from build123d import *

# Parameters (mm, degrees)
EXTRUDE_1_DEPTH     = 16.5
CUT_EXTRUDE_1_DEPTH = 89.239730281
SKETCH_3_R          = 3
CUT_EXTRUDE_2_DEPTH = 33


with BuildPart() as part:
    # 草圖1 → 填料-伸長1 (new, symmetric)
    with BuildSketch(Plane.XY):
        Polygon((0, 0), (85, 0), (85, 10), (78, 10), (78, 17), (75.5, 17), (75.5, 23), (63.5, 23), (63.5, 17), (61, 17), (61, 10), (50, 10), (50, 6), (0, 6), align=None)
    extrude(amount=EXTRUDE_1_DEPTH, both=True)

    # 草圖2 → 除料-伸長1 (cut, through all)
    with BuildSketch(Plane(origin=(0, 6, 0), x_dir=(1, 0, 0), z_dir=(0, 1, 0))):
        with BuildLine():
            Line((10, 4), (45, 4))
            ThreePointArc((45, 4), (49, 0), (45, -4))
            Line((45, -4), (10, -4))
            ThreePointArc((10, -4), (6, 0), (10, 4))
        make_face()
    extrude(amount=-CUT_EXTRUDE_1_DEPTH, mode=Mode.SUBTRACT)

    # 草圖3 → 除料-伸長2 (cut)
    with BuildSketch(Plane(origin=(78, 0, 0), x_dir=(0, 0, -1), z_dir=(1, 0, 0))):
        with Locations(Location((-10, 15, 0), (0, 0, 41.810314896))):
            Circle(SKETCH_3_R)
        with Locations(Location((10, 15, 0), (0, 0, 41.810314896))):
            Circle(SKETCH_3_R)
    extrude(amount=-CUT_EXTRUDE_2_DEPTH, mode=Mode.SUBTRACT)


solid = part.part
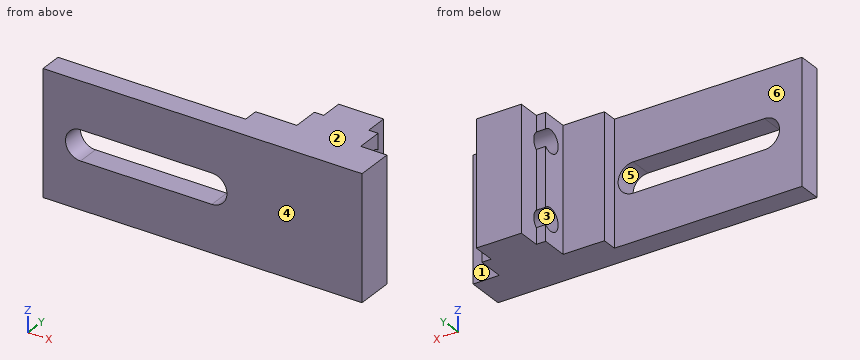
Can you work these out from the model? Positions are in its coordinate system, mm. Face numbers are marked on the shaded views. A direction names the side the tool comes from. Round coordinates to 2 decimals unless told otherwise and drop trailing zeros. Order: outer loops, then holes, each group sorted by start corner. A loop starts at its lowest first (then second) coordinate and runs counter-clockwise, first axis right, second up. Notation, with made-up numbers: (-9.75, 20.5) - (2.25, 20.5) arc R31 ccw to (2.25, 54.5) - close; hole circle Ø2 at (57, -8.75). An arc over 180 degrees is marked (long way). Answer in a Markdown table with one row per item.
(1) Suppose I cut it at B-B, the plane x = 14. Please give me the cut outline in (y, z).
From the geometry:
| item | result |
|---|---|
| outline | (0, -16.5) - (6, -16.5) - (6, -4) - (0, -4) - close; (0, 4) - (6, 4) - (6, 16.5) - (0, 16.5) - close |
(2) Suppose I cut it at A-A, the plane z = -10. Please give me the cut outline in (x, y), plus the area to 3 significant figures.
From the geometry:
| item | result |
|---|---|
| outline | (0, 0) - (85, 0) - (85, 10) - (78, 10) - (78, 12) - (61, 12) - (61, 10) - (50, 10) - (50, 6) - (0, 6) - close; (63.5, 18) - (75.5, 18) - (75.5, 23) - (63.5, 23) - close |
| area | 744 mm2 |
(3) Suppose I cut it at D-D, the plane x = 70.5. Please give me the cut outline in (y, z), plus the area to 3 significant figures.
From the geometry:
| item | result |
|---|---|
| outline | (0, -16.5) - (23, -16.5) - (23, 16.5) - (0, 16.5) - close; hole circle Ø6 at (15, -10); hole circle Ø6 at (15, 10) |
| area | 702 mm2 |
(4) Suppose I cut it at C-C, the plane y = 15. Please give me the cut outline in (x, z), plus the area to 3 significant figures.
From the geometry:
| item | result |
|---|---|
| outline | (61, -16.5) - (78, -16.5) - (78, -13) - (61, -13) - close; (61, -7) - (78, -7) - (78, 7) - (61, 7) - close; (61, 13) - (78, 13) - (78, 16.5) - (61, 16.5) - close |
| area | 357 mm2 |
(5) Please list where these lines run through material, in increasing order: L1, parallel to Z at x = 65, y = 15; L2, parallel to Y at x = 68, z = 10; L3, parallel to Z at x = 15, y = 5.25. Write a range as from..to.
From the geometry:
| item | result |
|---|---|
| L1 | z = -16.5..-13, -7..7, 13..16.5 |
| L2 | y = 0..12, 18..23 |
| L3 | z = -16.5..-4, 4..16.5 |
(6) Which directions (+Z, -Z, +X, -X, +Y, -Y) give clear straight access to the entire face, cutting with the end or side of a thin tool? Please do the marked faces 4, 5 and 6.
From the geometry:
| item | result |
|---|---|
| face 4 | +Z, -Z, +X, -X, -Y |
| face 5 | +Y, -Y |
| face 6 | +Z, -Z, -X, +Y |
(7) If we mould it in two halves opening along Y, with no side actions, what happens to the marked faces 1, 2 and 3? For each: released by +Y, released by -Y, zero draft, split by the parting line, or undercut.
From the geometry:
| item | result |
|---|---|
| face 1 | released by +Y |
| face 2 | zero draft |
| face 3 | undercut |
(8) For P1, Ø4, axis at y = 14, z = 2.5, coming from the -X side; P2, Ø12, axis at x = 56.5, z = 7.5, coming from the +Y side; P3, Ø4, axis at x = 11.5, z = -4.5, coming from the +Y side; P4, Ø8, axis at x = 15, y = 12, coming from the +Z side, each with a flat end and sliding along its axis, tell me the tip position at first contact or that it passes through.
From the geometry:
| item | result |
|---|---|
| P1 | stops at x = 61 |
| P2 | stops at y = 17 |
| P3 | stops at y = 6 |
| P4 | passes through |
